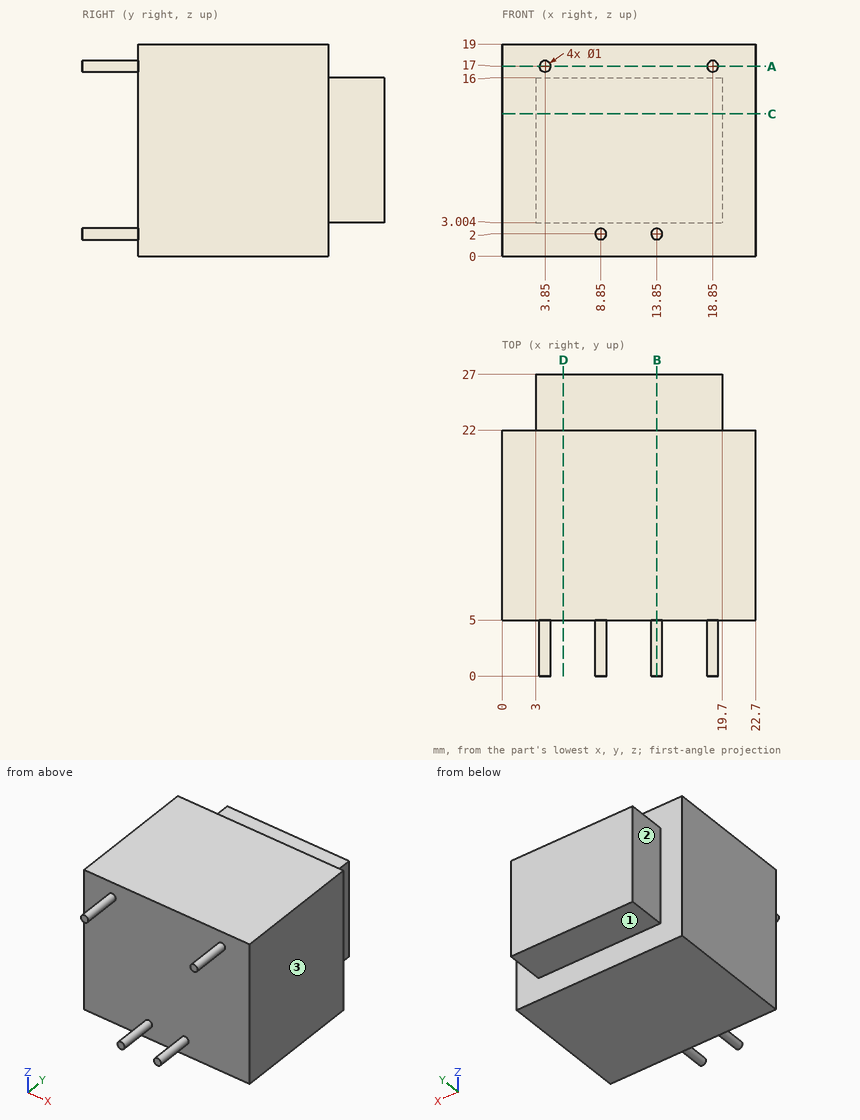
Check sheet for the drawn part. Datum: minimum x, y, z corner. Units: mm. A direction names the side the tool comes from. Round coordinates to 2 decimals unless told otherwise and drop trailing zeros. Loops run counter-clockwise (first coordinate to the right, second up) from the corner with the lowest first, then second, coordinate; pieces in that order, holes last. Notation, with made-up numbers: M -17,-27.5 L 20,-27.5 A26 ccw 20,6.5 Z; hole C -34,28 d3. An arc over 180 degrees is marked long. Write each question's results on one line, items separated by ' | '.
1) Scan lines: L1, parallel to Y at x = 2.5, z = 2; L2, parallel to Z at x = 16.5, y = 23; L3, parallel to Y at x = 11, z = 9. Record each from-to range of solid material in increasing order. Write a range as from..to.
Checks:
L1: y = 5..22 | L2: z = 3..16 | L3: y = 5..27
2) Access from +Z, -Z, +X, -X, +Y, -Y to the whole of each face (thin tool, end or side, straight path). Record for the marked faces 1, 2 and 3.
Checks:
face 1: -Z, +X, -X, +Y | face 2: +Z, -Z, -X, +Y | face 3: +Z, -Z, +X, +Y, -Y
3) Section check A-A on z = 17. Record the boundary of the cut face in (x, y).
Checks:
outline: M 0,5 L 3.35,5 L 3.35,0 L 4.35,0 L 4.35,5 L 18.35,5 L 18.35,0 L 19.35,0 L 19.35,5 L 22.7,5 L 22.7,22 L 0,22 Z
4) Section check B-B on x = 13.85. Record the boundary of the cut face in (y, z), then the cut area to 3 significant figures.
Checks:
outline: M 0,1.5 L 5,1.5 L 5,0 L 22,0 L 22,3 L 27,3 L 27,16 L 22,16 L 22,19 L 5,19 L 5,2.5 L 0,2.5 Z | area: 393 mm2
5) Section check D-D on x = 5.5. Record the boundary of the cut face in (y, z), then the cut area to 3 significant figures.
Checks:
outline: M 5,0 L 22,0 L 22,3 L 27,3 L 27,16 L 22,16 L 22,19 L 5,19 Z | area: 388 mm2
6) Gauge pin test, flat ends, axial feed: P1, Ø5.5, axis at x = 9.5, y = 25, coming from the +Z side; P2, Ø1.5, axis at y = 24.5, z = 6.5, coming from the +X side; P3, Ø5.5, axis at x = 8, z = 9.5, coming from the -Y side. Record the tip position at first contact, or that the pin passes through.
Checks:
P1: stops at z = 16 | P2: stops at x = 19.7 | P3: stops at y = 5
7) Section check C-C on z = 12.75. Record the boundary of the cut face in (x, y).
Checks:
outline: M 0,5 L 22.7,5 L 22.7,22 L 19.7,22 L 19.7,27 L 3,27 L 3,22 L 0,22 Z
